Autodesk Inventor part; units mm, degrees
ref_plane "YZ Plane" through (0, 0, 0) normal (1, 0, 0) x (0, 1, 0)
ref_plane "XZ Plane" through (0, 0, 0) normal (0, 1, 0) x (-1, 0, 0)
ref_plane "XY Plane" through (0, 0, 0) normal (0, 0, 1) x (1, 0, 0)
sketch "Sketch1" plane through (0, 0, 0) normal (0, 0, 1) x (1, 0, 0)
  line L0 (-16, 12.5) -> (-13, 12.5)
  line L1 (-13, 12.5) -> (-13, -9.5)
  line L2 (-13, -9.5) -> (13, -9.5)
  line L3 (13, -9.5) -> (13, 12.5)
  line L4 (13, 12.5) -> (16, 12.5)
  line L5 (16, 12.5) -> (16, -12.5)
  line L6 (16, -12.5) -> (-16, -12.5)
  line L7 (-16, -12.5) -> (-16, 12.5)
  point P0 (0, 0)
  dimension "d0" = 3
  dimension "d2" = 3
  dimension "d3" = 25
  dimension "d4" = 32
  dimension "d5" = 16
  dimension "d7" = 12.5
  dimension "d8" = 3
  dimension "d95" = 25
extrude "Extrusion1" add sketch "Sketch1" against normal blind 558.8
sketch "Sketch7" plane through (-16, -12.5, 0) normal (0, -1, 0) x (1, 0, 0)
  line L0 (32, 0) -> (0, 0)
  line L1 (32, -558.8) -> (0, -558.8)
  line L2 (32, 0) -> (32, -558.8)
  circle A0 centre (16, -11) radius 3.175
  circle A1 centre (16, -547.8) radius 3.175
  point P0 (16, 0)
  dimension "d103" = 6.35
  dimension "d104" = 11
  dimension "d105" = 16
  dimension "d106" = 6.35
  dimension "d108" = 16
  dimension "d109" = 11
hole "Hole3" at (0, -12.5, -547.8) at (0, -12.5, -11) direction (0, 1, 0) diameter 6.35 end through all
sketch "Sketch8" plane through (-16, -12.5, 0) normal (0, -1, 0) x (1, 0, 0)
  line L0 (26.7, -35.2242) -> (48.3, -35.2242) construction
  arc A0 (26.7, -276.4246) -> (26.7, -282.7746) centre (26.7, -279.5996) ccw construction
  line L1 (26.7, -276.4246) -> (48.3, -276.4246) construction
  arc A1 (48.3, -282.7746) -> (48.3, -276.4246) centre (48.3, -279.5996) ccw construction
  line L2 (48.3, -282.7746) -> (26.7, -282.7746) construction
  arc A2 (26.7, -155.8244) -> (26.7, -162.1744) centre (26.7, -158.9994) ccw construction
  line L3 (26.7, -155.8244) -> (48.3, -155.8244) construction
  arc A3 (48.3, -162.1744) -> (48.3, -155.8244) centre (48.3, -158.9994) ccw construction
  line L4 (48.3, -162.1744) -> (26.7, -162.1744) construction
  arc A4 (48.3, -523.975) -> (48.3, -517.625) centre (48.3, -520.8) ccw construction
  line L5 (48.3, -523.975) -> (26.7, -523.975) construction
  arc A5 (26.7, -517.625) -> (26.7, -523.975) centre (26.7, -520.8) ccw construction
  line L6 (26.7, -517.625) -> (48.3, -517.625) construction
  arc A6 (26.7, -397.0248) -> (26.7, -403.3748) centre (26.7, -400.1998) ccw construction
  line L7 (26.7, -397.0248) -> (48.3, -397.0248) construction
  arc A7 (48.3, -403.3748) -> (48.3, -397.0248) centre (48.3, -400.1998) ccw construction
  line L8 (48.3, -403.3748) -> (26.7, -403.3748) construction
  arc A8 (48.3, -41.5742) -> (48.3, -35.2242) centre (48.3, -38.3992) ccw construction
  line L9 (48.3, -41.5742) -> (26.7, -41.5742) construction
  arc A9 (26.7, -35.2242) -> (26.7, -41.5742) centre (26.7, -38.3992) ccw construction
  line L10 (26.7, -35.2242) -> (48.3, -35.2242) construction
  line L11 (61, -22.3992) -> (14, -22.3992) construction
  line L12 (14, -22.3992) -> (14, -536.8) construction
  line L13 (61, -536.8) -> (14, -536.8) construction
  line L14 (61, -22.3992) -> (61, -536.8) construction
  circle A10 centre (26.7, -38.3992) radius 3.175
  circle A11 centre (26.7, -158.9994) radius 3.175
  circle A12 centre (26.7, -279.5996) radius 3.175
  circle A13 centre (26.7, -400.1998) radius 3.175
  circle A14 centre (26.7, -520.8) radius 3.175
  point P0 (16, 0)
hole "Hole4" at (10.7, -12.5, -38.3992) at (10.7, -12.5, -158.9994) at (10.7, -12.5, -279.5996) at (10.7, -12.5, -400.1998) at (10.7, -12.5, -520.8) direction (0, 1, 0) diameter 6.35 depth 3 tip angle 118
equation "\"d2\" = d0"
equation "\"d8\" = d0"
equation "\"d95\" = d3"
properties part number "26in C-Channel Left" material "Aluminum 6061"
Model file for the job. Use its own axes, mm. A direction names the side the tool comes from. Coordinates: 2 decimals unless noted, no trailing zeros. Order: outer loops, then holes, each group sorted by start corner. A loop starts at its lowest first (then second) coordinate and runs counter-clockwise, first axis right, second up. Notation, with made-up numbers: (34.25, 33) -> (48.25, 33) arc R17 ccw to (48.25, 66) -> close; hole circle Ø8 at (19.25, 29). An arc over 180 degrees is marked (long way). Return JSON: item names as keys, results as strings.
Item 1: Mould opens along X. For faces 1 (the face through (-13, 2, -275)), 2 (the face through (-1, -10, 0)), 3 (the face through (0, -9.5, -275)), 4 (the face through (16, 0, -275)) say: pulls with the +X half, pulls with the -X half, needs draft (parallel to the pull), parting line crosses it, or undercut.
Model answer:
{"face 1": "undercut", "face 2": "needs draft", "face 3": "undercut", "face 4": "pulls with the +X half"}
Item 2: Slice it at C-C (x = -8). Write the cut outline in (y, z), then the cut area to 3 significant figures.
Model answer:
{"outline": "(-12.5, -558.8) -> (-9.5, -558.8) -> (-9.5, 0) -> (-12.5, 0) -> close", "area": "1,680 mm²"}
Item 3: Wall check: line 1 along Z through (x, y) = (0, -10.85) (3 decimals); line 2 along Z through (x, y) = (10.7, -11.9) (3 decimals); line 3 along X through (y, z) = (-6, -59). Give the ranges that are in metal, low to high. Write a range as from..to.
Model answer:
{"line 1": "z = -558.8..-550.975, -544.625..-14.175, -7.825..0", "line 2": "z = -558.8..-523.975, -517.625..-403.375, -397.025..-282.775, -276.425..-162.174, -155.824..-41.574, -35.224..0", "line 3": "x = -16..-13, 13..16"}
Item 4: 3-axis set-ups, long thin cutter, end or side, ignore diameter. For faces 5 (the face through (13, 1, -275)), 6 (the face through (-1, -10, -558.8)): which of +Z, -Z, +X, -X, +Y, -Y reach the whole face in a straight line?
Model answer:
{"face 5": "+Z, -Z, +Y", "face 6": "-Z, +X, -X, +Y, -Y"}
Item 5: Pin check, flat tip, straight feed: P1, Ø8, axis at x = 3.5, z = -204, coming from the +Y side. Stop position of the tip, or through.
Model answer:
{"P1": "stops at y = -9.5"}
Item 6: Slice it at A-A (y = 2.25). Write the cut outline in (x, z).
Model answer:
{"outline": "(-16, -558.8) -> (-13, -558.8) -> (-13, 0) -> (-16, 0) -> close; (13, -558.8) -> (16, -558.8) -> (16, 0) -> (13, 0) -> close"}
Item 7: Slice it at B-B (z = -99.5). Write the cut outline in (x, y).
Model answer:
{"outline": "(-16, -12.5) -> (16, -12.5) -> (16, 12.5) -> (13, 12.5) -> (13, -9.5) -> (-13, -9.5) -> (-13, 12.5) -> (-16, 12.5) -> close"}
